from build123d import *

# Parameters (mm, degrees)
F1_DEPTH = 25


with BuildPart() as f1:
    # F0 (on Front) → F1 (new body)
    with BuildSketch(Plane.XZ):
        with BuildLine():
            ThreePointArc((13.51559, -9.3768), (83.224894, -26.042828), (150, 0))
            ThreePointArc((150, 0), (83.224894, 26.042828), (13.51559, 9.3768))
            ThreePointArc((13.51559, 9.3768), (6.596932, 4.920265), (0, 0))
            ThreePointArc((0, 0), (6.596932, -4.920265), (13.51559, -9.3768))
        make_face()
        with BuildLine():
            ThreePointArc((0, 0), (6.596932, 4.920265), (13.51559, 9.3768))
            Line((13.51559, 9.3768), (-9.007419, 28.40198))
            ThreePointArc((-9.007419, 28.40198), (-20.734502, 27.33708), (-19.515619, 15.625))
            Line((-19.515619, 15.625), (0, 0))
        make_face()
        with BuildLine():
            Line((-9.007419, -28.40198), (13.51559, -9.3768))
            ThreePointArc((13.51559, -9.3768), (6.596932, -4.920265), (0, 0))
            Line((0, 0), (-19.515619, -15.625))
            ThreePointArc((-19.515619, -15.625), (-20.734502, -27.33708), (-9.007419, -28.40198))
        make_face()
    extrude(amount=F1_DEPTH)


solid = f1.part
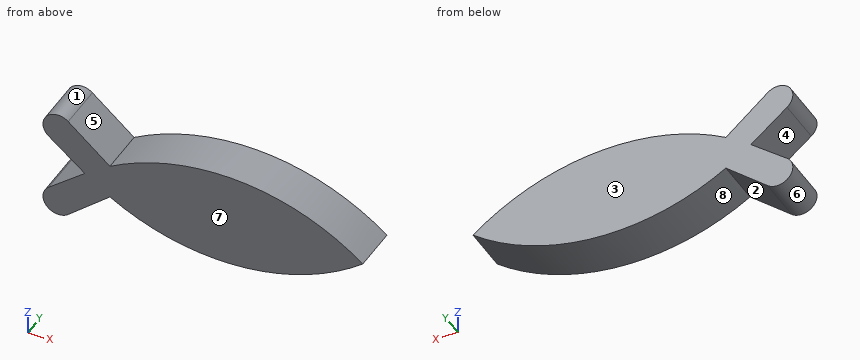
Design review of the part built by this model. Coordinates are the model's own, in mm. Face numbers are marked on the shaded views. A direction names the side the tool comes from. Coordinates: 2 decimals unless noted, no trailing zeros. Order: outer loops, then holes, each group sorted by start corner. A loop starts at its lowest first (then second) coordinate and runs counter-clockwise, first axis right, second up. Notation, with made-up numbers: (-1.5, 62.25) -> (28.5, 62.25) arc R22 ccw to (28.5, 90.25) -> close; hole circle Ø7 at (82.25, 6.25). An arc over 180 degrees is marked (long way). One line per item, written item: value.
1) To check wall thickness, follow probe 1 along X at (y, z) = (-17.75, 9.5); probe 2 along Z at (x, y) = (-9.5, -18); probe 3 along Z at (x, y) = (13.5, -10.5). State the ranges of each line that lie inside material, in increasing order. Write a range as [from, to].
Output values:
probe 1: x = [-11.87, 13.37], [13.72, 136.28]
probe 2: z = [-28.79, -7.61], [7.61, 28.79]
probe 3: z = [-9.39, 9.39]
2) We need section C-C, the plane x = -2. Give the boundary of the cut face in (y, z).
Output values:
outline: (-25, -22.48) -> (0, -22.48) -> (0, -1.6) -> (-25, -1.6) -> close; (-25, 1.6) -> (0, 1.6) -> (0, 22.48) -> (-25, 22.48) -> close
3) Clearance check with flat-ended pins moving along their axes: P1, Ø4, axis at x = 74, y = -7.5, coming from the -Z side; P2, Ø12, axis at x = 87, y = -21, coming from the -Z side; P3, Ø6, axis at x = 77.5, y = -10, coming from the +Z side. State where each tip first meets the part, or that it passes through.
Output values:
P1: stops at z = -26.33
P2: stops at z = -26.17
P3: stops at z = 26.33
4) We need section D-D, the plane z = 6. Give the boundary of the cut face in (x, y), then the cut area to 3 significant figures.
Output values:
outline: (-7.49, -25) -> (141.82, -25) -> (141.82, 0) -> (-7.49, 0) -> close
area: 3,730 mm2
5) Draft analysis for pull direction X (two halves, no side actions). For the marked faces 6, 7 and 8, state which applies: +X half, -X half, draft (parallel to the pull), parting line (faces both ways), or undercut.
Output values:
face 6: parting line
face 7: draft
face 8: undercut
6) Machinability: for the marked faces 1, 2, 3, 4 and 5, which of the approach directions +Z, -Z, +X, -X, +Y, -Y give a long, thin tool a straight path to every point of the face, cutting with its end or side? Answer none if there is none.
Output values:
face 1: +Y, -Y
face 2: -Z, +Y, -Y
face 3: +Z, -Z, +X, -X, +Y
face 4: -X, +Y, -Y
face 5: +Z, +Y, -Y
7) We need section B-B, the plane y = -5.25. Give the boundary of the cut face in (x, z) (1 decimal), then the cut area to 3 significant figures.
Output values:
outline: (-19.5, -15.6) arc R8.3 ccw (long way) to (-9, -28.4) -> (13.5, -9.4) arc R120 ccw to (150, 0) arc R120 ccw to (13.5, 9.4) -> (-9, 28.4) arc R8.3 ccw (long way) to (-19.5, 15.6) -> (0, 0) -> close
area: 6,490 mm2
8) We need section A-A, the plane z = 24.5. Give the boundary of the cut face in (x, y).
Output values:
outline: (-22.26, -25) -> (-4.39, -25) -> (-4.39, 0) -> (-22.26, 0) -> close; (54.15, -25) -> (95.85, -25) -> (95.85, 0) -> (54.15, 0) -> close
